```python
from build123d import *

# Parameters (mm, degrees)
F0_W          = 152.4
F0_H          = 76.2
F1_DEPTH      = 3.175
F2_W          = 117.475
F2_H          = 66.675
F3_DEPTH      = 9.525
F4_W          = 114.3
F4_H          = 63.5
F5_DEPTH      = 11.1125
F6_W          = 50.8
F6_H          = 9.525
F7_DEPTH      = 25.4
F7_DEPTH_BACK = 25.4
F8_R          = 1.5875
F9_DEPTH      = 25.4


with BuildPart() as f1:
    # F0 (on Top) → F1 (new body)
    with BuildSketch(Plane.XY):
        with Locations((-2.3664589537, 0)):
            Rectangle(F0_W, F0_H)
    extrude(amount=F1_DEPTH)

    # F2 (on face) → F3 (join)
    with BuildSketch(Plane.XY.offset(3.175)):
        Rectangle(F2_W, F2_H)
    extrude(amount=F3_DEPTH)

    # F4 (on face) → F5 (cut)
    with BuildSketch(Plane(origin=(0, 0, 0), x_dir=(1, 0, 0), z_dir=(0, 0, -1))):
        Rectangle(F4_W, F4_H)
    extrude(amount=-F5_DEPTH, mode=Mode.SUBTRACT)

    # F6 (on face) → F7 (cut, two sides)
    with BuildSketch(Plane(origin=(-58.7375, 0, 0), x_dir=(0, -1, 0), z_dir=(-1, 0, 0))) as f7_sk:
        with Locations((0, 4.7625)):
            Rectangle(F6_W, F6_H)
    extrude(amount=-F7_DEPTH, mode=Mode.SUBTRACT)
    extrude(f7_sk.sketch, amount=F7_DEPTH_BACK, mode=Mode.SUBTRACT)

    # F8 (on face) → F9 (cut)
    with BuildSketch(Plane.XY.offset(3.175)):
        with Locations((-72.2164589537, 31.75)):
            Circle(F8_R)
        with Locations((-72.2164589537, -31.75)):
            Circle(F8_R)
        with Locations((67.4835410463, 31.75)):
            Circle(F8_R)
        with Locations((67.4835410463, -31.75)):
            Circle(F8_R)
    extrude(amount=-F9_DEPTH, mode=Mode.SUBTRACT)


solid = f1.part
```
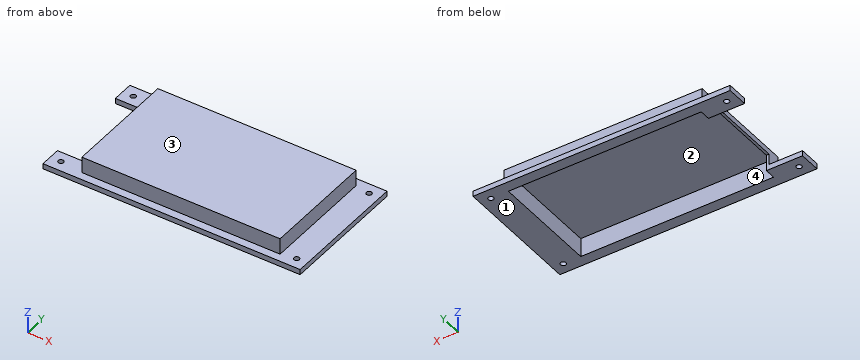
Geometry: final body of the model. Coordinates: model frame, mm. Face numbers are marked on the shaded views. A direction names the side the tool comes from. Coordinates: 2 decimals unless noted, no trailing zeros. Loops run counter-clockwise (first coordinate to the right, second up) from the corner with the lowest first, then second, coordinate; pieces in that order, holes last. Notation, with made-up numbers: (1, 25) -> (59, 25) arc R22 ccw to (59, 44) -> close; hole circle Ø10 at (51.5, -4.5). An arc over 180 degrees is marked (long way). Use a Markdown table: item, result. Add a question column.
(1) Section query C-C, the plane z = 6. Return loops of the section in (x, y), plus the area to 3 significant figures.
(2) Mould query, pull axis X, two halves, no side actions, for the marked faces 3 and 4. Classes: pulls with the +X half, pulls with the -X half, needs draft (parallel to the pull), parting line crosses it, or undercut.
(3) Access query for the marked faces 1 and 2. Directions: +Z, -Z, +X, -X, +Y, -Y. A direction counts if a zero-diameter tool reaches every point of the face in a straight line with its end or side. Return the directions, or none.
(4) Pin query (flat end, axial travel): pin 1 Ø1.5 at (x, y) = (9.5, -18.5) entering from -Z; pin 2 Ø4 at (y, z) = (0, 2) entering from -X; pin 3 Ø3.5 at (x, y) = (-72.22, 31.75) entering from +Z (3 decimals); pin 4 Ø2.5 at (x, y) = (67.48, -31.75) entering from +Z. Return the tip coordinate at first contact, or that it passes through.
(5) Line query: line 1 along Y through (x, z) = (52, 2.5); line 2 along Y through (x, z) = (-56.5, 6.5); line 3 along Z through (x, y) = (67.5, 9.5) (3 decimals). Output: solid intervals per line, ascending.
Answer:
| question | item | result |
|---|---|---|
| 1 | outline | (-58.74, -33.34) -> (58.74, -33.34) -> (58.74, 33.34) -> (-58.74, 33.34) -> (-58.74, 25.4) -> (-57.15, 25.4) -> (-57.15, 31.75) -> (57.15, 31.75) -> (57.15, -31.75) -> (-57.15, -31.75) -> (-57.15, -25.4) -> (-58.74, -25.4) -> close |
| 1 | area | 494 mm^2 |
| 2 | face 3 | needs draft |
| 2 | face 4 | undercut |
| 3 | face 1 | -Z, +X, -X, +Y, -Y |
| 3 | face 2 | -Z |
| 4 | pin 1 | stops at z = 11.11 |
| 4 | pin 2 | stops at x = 57.15 |
| 4 | pin 3 | stops at z = 3.175 |
| 4 | pin 4 | passes through |
| 5 | line 1 | y = -38.1 to -31.75, 31.75 to 38.1 |
| 5 | line 2 | y = -33.34 to -31.75, 31.75 to 33.34 |
| 5 | line 3 | z = 0 to 3.175 |
